from build123d import *

# Parameters (mm, degrees)
SM_BASE_FLANGE_1_DEPTH   = 41
SKETCH_9_R               = 2
CUT_EXTRUDE_4_DEPTH      = 69.441580929
CUT_EXTRUDE_5_DEPTH      = 83.772277968
CUT_EXTRUDE_5_DEPTH_BACK = 83.772277968
SKETCH_10_R              = 2.5


# Sheet-metal steps are written as plain solids
with BuildPart() as part:
    # Sketch 1 → Базовая кромка1 (new body)
    with BuildSketch(Plane.XY):
        with BuildLine():
            Line((-25, 42.5), (-25, 1))
            ThreePointArc((-25, 1), (-24.707106781, 0.292893219), (-24, 0))
            Line((-24, 0), (24, 0))
            ThreePointArc((24, 0), (24.707106781, 0.292893219), (25, 1))
            Line((25, 1), (25, 42.5))
            Line((25, 42.5), (29, 42.5))
            Line((29, 42.5), (29, 1))
            ThreePointArc((29, 1), (27.535533906, -2.535533906), (24, -4))
            Line((24, -4), (-24, -4))
            ThreePointArc((-24, -4), (-27.535533906, -2.535533906), (-29, 1))
            Line((-29, 1), (-29, 42.5))
            Line((-29, 42.5), (-25, 42.5))
        make_face()
    extrude(amount=SM_BASE_FLANGE_1_DEPTH)

    # Эскиз9 → Вырез-Вытянуть4 (cut, through all)
    with BuildSketch(Plane.XZ.offset(4)):
        with Locations((0, 5)):
            Circle(SKETCH_9_R)
        with Locations((-13.423393759, 12.75)):
            Circle(SKETCH_9_R)
        with Locations((-13.423393759, 28.25)):
            Circle(SKETCH_9_R)
        with Locations((0, 36)):
            Circle(SKETCH_9_R)
        with Locations((13.423393759, 28.25)):
            Circle(SKETCH_9_R)
        with Locations((13.423393759, 12.75)):
            Circle(SKETCH_9_R)
    extrude(amount=-CUT_EXTRUDE_4_DEPTH, mode=Mode.SUBTRACT)

    # Эскиз10 → Вырез-Вытянуть5 (cut, two sides: drawn at the far end of the back side and taken through both)
    with BuildSketch(Plane(origin=(29, 0, 0), x_dir=(0, 0, -1), z_dir=(1, 0, 0)).offset(-CUT_EXTRUDE_5_DEPTH_BACK)):
        with Locations((-33, 25)):
            Circle(SKETCH_10_R)
        with Locations((-20.5, 25)):
            Circle(SKETCH_10_R)
        with Locations((-8, 25)):
            Circle(SKETCH_10_R)
        with Locations((-20.5, 12.5)):
            Circle(SKETCH_10_R)
        with Locations((-20.5, 37.5)):
            Circle(SKETCH_10_R)
    extrude(amount=CUT_EXTRUDE_5_DEPTH + CUT_EXTRUDE_5_DEPTH_BACK, mode=Mode.SUBTRACT)


solid = part.part
Read the model definition and answer for the solid it produces. Units are mm, in the model's axes. A direction names the side the tool comes from. Round coordinates to 2 decimals unless told otherwise and drop trailing zeros. Write each loop counter-clockwise with the first axis right and the second up, starting at its lowest first coordinate (ties: lowest second). Pieces come first, ordered by that corner, then holes.
1. Determine the mould class of faces 1 (the face through (29, 22, 20)), 2 (the face through (27, 42.5, 20)), 3 (the face through (25, 21, 20)) for opening direction X: pulls with the +X half, pulls with the -X half, needs draft (parallel to the pull), parting line crosses it, or undercut.
2. The part is cut by section D-D, the plane y = 37.5. Determine the outline of the cut face in (x, z).
3. The part is cut by section B-B, the plane y = 16. Determine the outline of the cut face in (x, z), then the cut area to 3 significant figures.
4. Which of the six approach directions +Z, -Z, +X, -X, +Y, -Y give full straight-line access (tool end or side, diameter ignored) to faces 4 (the face through (0, 0, 20)), 5 (the face through (26.97, 27.48, 33.33))?
5. Given pin 1 Ø6 at (y, z) = (25, 33) entering from -X; pin 2 Ø4.5 at (y, z) = (12.5, 20.5) entering from -X; pin 3 Ø6.5 at (x, z) = (0, 36) entering from +Y, each flat-ended and moving along its own axis, determine where each tip first touches the part or whether it passes through.
6. The part is cut by section C-C, the plane x = 0. Determine the outline of the cut face in (y, z).
7. The part is cut by section A-A, the plane z = 8. Determine the outline of the cut face in (x, y).
8. Straight lines are drawn through the part: L1, parallel to Z at x = 26, y = 25; L2, parallel to Z at x = 0, y = -2.45; L3, parallel to X at y = 9, z = 23. For each, find the intervals that lie inside material, in ascending order.
Values:
1. face 1: pulls with the +X half
1. face 2: needs draft
1. face 3: undercut
2. outline: (-29, 0) - (-25, 0) - (-25, 18) - (-29, 18) - close; (-29, 23) - (-25, 23) - (-25, 41) - (-29, 41) - close; (25, 0) - (29, 0) - (29, 18) - (25, 18) - close; (25, 23) - (29, 23) - (29, 41) - (25, 41) - close
3. outline: (-29, 0) - (-25, 0) - (-25, 41) - (-29, 41) - close; (25, 0) - (29, 0) - (29, 41) - (25, 41) - close
3. area: 328 mm2
4. face 4: +Z, -Z, +Y
4. face 5: +X, -X
5. pin 1: stops at x = -29
5. pin 2: passes through
5. pin 3: stops at y = 0
6. outline: (-4, 0) - (0, 0) - (0, 3) - (-4, 3) - close; (-4, 7) - (0, 7) - (0, 34) - (-4, 34) - close; (-4, 38) - (0, 38) - (0, 41) - (-4, 41) - close
7. outline: (-29, 1) arc R5 ccw to (-24, -4) - (24, -4) arc R5 ccw to (29, 1) - (29, 22.5) - (25, 22.5) - (25, 1) arc R1 cw to (24, 0) - (-24, 0) arc R1 cw to (-25, 1) - (-25, 22.5) - (-29, 22.5) - close; (-29, 27.5) - (-25, 27.5) - (-25, 42.5) - (-29, 42.5) - close; (25, 27.5) - (29, 27.5) - (29, 42.5) - (25, 42.5) - close
8. L1: z = 0 to 5.5, 10.5 to 18, 23 to 30.5, 35.5 to 41
8. L2: z = 0 to 3, 7 to 34, 38 to 41
8. L3: x = -29 to -25, 25 to 29
